Read the model definition and answer for the solid it produces. Units are mm, in the model's axes. A direction names the side the tool comes from. Coordinates: 2 decimals unless noted, no trailing zeros. Order: outer loops, then holes, each group sorted by start corner. A loop starts at its lowest first (then second) coordinate and runs counter-clockwise, first axis right, second up. Notation, with made-up numbers: (6.5, -27.75) - (48.5, -27.75) arc R33 cw to (48.5, 8.25) - close; hole circle Ø1 at (57, 67). An arc over 180 degrees is marked (long way). Use one line per item in the form item = value.
```python
from build123d import *

# Parameters (mm, degrees)
F0_W     = 63.5
F0_H     = 35.56
F0_R     = 3.937
F0_R_2   = 11.303
F0_R_3   = 7.62
F0_R_4   = 5.08
F0_H_2   = 15.24
F0_H_3   = 38.1
F1_DEPTH = 19.05
F2_DEPTH = 76.2
F3_DEPTH = 3.175
F4_DEPTH = 6.35
F5_R     = 7.366
F6_DEPTH = 19.05
F7_DEPTH = 50.8
F8_DEPTH = 57.15


with BuildPart() as f1:
    # F0 (on Top) → F1 (new body)
    with BuildSketch(Plane.XY):
        with Locations((31.75, 17.78)):
            Rectangle(F0_W, F0_H)
        with Locations((31.75, 11.176)):
            Circle(F0_R, mode=Mode.SUBTRACT)
        with Locations((49.9618, 59.944)):
            Circle(F0_R_2)
        with Locations((49.9618, 59.944)):
            Circle(F0_R_3, mode=Mode.SUBTRACT)
        with Locations((13.5382, 59.944)):
            Circle(F0_R_2)
        with Locations((13.5382, 59.944)):
            Circle(F0_R_3, mode=Mode.SUBTRACT)
        with Locations((49.9618, 59.944)):
            Circle(F0_R_3)
        with Locations((49.9618, 59.944)):
            Circle(F0_R_4, mode=Mode.SUBTRACT)
        with Locations((13.5382, 59.944)):
            Circle(F0_R_3)
        with Locations((13.5382, 59.944)):
            Circle(F0_R_4, mode=Mode.SUBTRACT)
        with Locations((31.75, 81.28)):
            Rectangle(F0_W, F0_H_2)
        with Locations((11.43, 81.28)):
            Circle(F0_R, mode=Mode.SUBTRACT)
        with Locations((52.07, 81.28)):
            Circle(F0_R, mode=Mode.SUBTRACT)
        with Locations((31.75, 54.61)):
            Rectangle(F0_W, F0_H_3)
        with Locations((13.5382, 59.944)):
            Circle(F0_R_2, mode=Mode.SUBTRACT)
        with Locations((49.9618, 59.944)):
            Circle(F0_R_2, mode=Mode.SUBTRACT)
        with Locations((49.9618, 59.944)):
            Circle(F0_R_4)
        with Locations((13.5382, 59.944)):
            Circle(F0_R_4)
    extrude(amount=F1_DEPTH)

    # F0 (on Top) → F2 (join)
    with BuildSketch(Plane.XY):
        with Locations((31.75, 54.61)):
            Rectangle(F0_W, F0_H_3)
        with Locations((13.5382, 59.944)):
            Circle(F0_R_2, mode=Mode.SUBTRACT)
        with Locations((49.9618, 59.944)):
            Circle(F0_R_2, mode=Mode.SUBTRACT)
        with Locations((13.5382, 59.944)):
            Circle(F0_R_2)
        with Locations((13.5382, 59.944)):
            Circle(F0_R_3, mode=Mode.SUBTRACT)
        with Locations((49.9618, 59.944)):
            Circle(F0_R_2)
        with Locations((49.9618, 59.944)):
            Circle(F0_R_3, mode=Mode.SUBTRACT)
        with Locations((49.9618, 59.944)):
            Circle(F0_R_3)
        with Locations((49.9618, 59.944)):
            Circle(F0_R_4, mode=Mode.SUBTRACT)
        with Locations((13.5382, 59.944)):
            Circle(F0_R_3)
        with Locations((13.5382, 59.944)):
            Circle(F0_R_4, mode=Mode.SUBTRACT)
        with Locations((49.9618, 59.944)):
            Circle(F0_R_4)
        with Locations((13.5382, 59.944)):
            Circle(F0_R_4)
    extrude(amount=F2_DEPTH)

    # F0 (on Top) → F3 (cut)
    with BuildSketch(Plane.XY):
        with Locations((49.9618, 59.944)):
            Circle(F0_R_2)
        with Locations((49.9618, 59.944)):
            Circle(F0_R_3, mode=Mode.SUBTRACT)
        with Locations((13.5382, 59.944)):
            Circle(F0_R_2)
        with Locations((13.5382, 59.944)):
            Circle(F0_R_3, mode=Mode.SUBTRACT)
    extrude(amount=F3_DEPTH, mode=Mode.SUBTRACT)

    # F0 (on Top) → F4 (cut)
    with BuildSketch(Plane.XY):
        with Locations((49.9618, 59.944)):
            Circle(F0_R_3)
        with Locations((49.9618, 59.944)):
            Circle(F0_R_4, mode=Mode.SUBTRACT)
        with Locations((13.5382, 59.944)):
            Circle(F0_R_3)
        with Locations((13.5382, 59.944)):
            Circle(F0_R_4, mode=Mode.SUBTRACT)
    extrude(amount=F4_DEPTH, mode=Mode.SUBTRACT)

    # F5 (on face) → F6 (cut)
    with BuildSketch(Plane(origin=(0, 73.66, 0), x_dir=(-1, 0, 0), z_dir=(0, 1, 0))):
        with Locations((-49.9618, 57.15)):
            Circle(F5_R)
    extrude(amount=-F6_DEPTH, mode=Mode.SUBTRACT)

    # F5 (on face) → F7 (cut)
    with BuildSketch(Plane(origin=(0, 73.66, 0), x_dir=(-1, 0, 0), z_dir=(0, 1, 0))):
        with Locations((-13.5382, 57.15)):
            Circle(F5_R)
    extrude(amount=-F7_DEPTH, mode=Mode.SUBTRACT)

    # F0 (on Top) → F8 (cut)
    with BuildSketch(Plane.XY):
        with Locations((49.9618, 59.944)):
            Circle(F0_R_4)
        with Locations((13.5382, 59.944)):
            Circle(F0_R_4)
    extrude(amount=F8_DEPTH, mode=Mode.SUBTRACT)


solid = f1.part
```
(1) Straight lines are drawn through the part: L1, parallel to X at y = 59, z = 38; L2, parallel to Y at x = 49.5, z = 45; L3, parallel to Y at x = 58.5, z = 49. For each, find the intervals that lie inside material, in ascending order.
Answer list:
L1 = 0 to 8.55, 18.53 to 44.97, 54.95 to 63.5
L2 = 35.56 to 54.89, 65 to 73.66
L3 = 35.56 to 73.66
(2) Section C-C, the plane y = 81.28 is taken. Write down the section's boundary in (x, z).
Answer list:
outline = (0, 0) - (7.49, 0) - (7.49, 19.05) - (0, 19.05) - close; (15.37, 0) - (48.13, 0) - (48.13, 19.05) - (15.37, 19.05) - close; (56.01, 0) - (63.5, 0) - (63.5, 19.05) - (56.01, 19.05) - close
(3) Section A-A, the plane z = 57.15 is taken. Write down the section's boundary in (x, y), then the cut area to 3 significant figures.
Answer list:
outline = (0, 35.56) - (6.17, 35.56) - (6.17, 73.66) - (0, 73.66) - close; (20.9, 35.56) - (63.5, 35.56) - (63.5, 73.66) - (57.33, 73.66) - (57.33, 54.61) - (42.6, 54.61) - (42.6, 73.66) - (20.9, 73.66) - close
area = 1,580 mm2
(4) The mould has two halves that part along Z. Classify faces 5 (the flat face through (52, 55, 6.35)), 6 (the cylindrical face through (50.921, 64.268, 64.453)), 7 (the cylindrical face through (14.497, 54.877, 64.453)), 8 (the flat face through (31, 18, 19.05)): +Z half, -Z half, draft (parallel to the pull), parting line (faces both ways), or undercut.
Answer list:
face_5 = -Z half
face_6 = undercut
face_7 = undercut
face_8 = +Z half
(5) Section B-B, the plane x = 31.75 is taken. Write down the section's boundary in (y, z), then the cut area to 3 significant figures.
Answer list:
outline = (0, 0) - (7.24, 0) - (7.24, 19.05) - (0, 19.05) - close; (15.11, 0) - (88.9, 0) - (88.9, 19.05) - (73.66, 19.05) - (73.66, 76.2) - (35.56, 76.2) - (35.56, 19.05) - (15.11, 19.05) - close
area = 3,720 mm2
(6) Which of the six approach directions +Z, -Z, +X, -X, +Y, -Y give full straight-line access (tool end or side, diameter ignored) to faces 1 (the flat face through (31, 55, 76.2)), 2 (the cylindrical face through (12.55, 67.5, 4.74)), 3 (the flat face through (31, 73.66, 47)), 4 (the flat face through (31, 35.56, 47))?
Answer list:
face_1 = +Z, +X, -X, +Y, -Y
face_2 = -Z
face_3 = +Z, +X, -X, +Y
face_4 = +Z, +X, -X, -Y
(7) Given pin 1 Ø19 at (x, z) = (13.54, 57.15) entering from +Y; pin 2 Ø10 at (x, y) = (54.5, 10.5) entering from +Z; pin 3 Ø4.5 at (x, y) = (11.5, 60.5) entering from -Z; pin 4 Ø4 at (y, z) = (24, 22.5) entering from -X, each flat-ended and moving along its own axis, determine where each tip first touches the part or whether it passes through.
Answer list:
pin_1 = 73.66
pin_2 = 19.05
pin_3 = 63.14
pin_4 = through
(8) Section D-D, the plane y = 43.5 is taken. Write down the section's boundary in (x, z).
Answer list:
outline = (0, 0) - (63.5, 0) - (63.5, 76.2) - (0, 76.2) - close; hole circle Ø14.73 at (13.54, 57.15)
